Geometry check sheet. Reference: drawing and pictorial views, mm from the part's lowest x, y, z. A direction names the side the tool comes from. Round coordinates to 2 decimals unless told otherwise and drop trailing zeros. Loops run counter-clockwise (first coordinate to the right, second up) from the corner with the lowest first, then second, coordinate; pieces in that order, holes last. Notation, with made-up numbers: (-35.5, -29.75) -> (-1.5, -29.75) arc R20 cw to (-1.5, -14.75) -> close; hole circle Ø2 at (53, -25). An arc over 180 degrees is marked (long way). Use one line per item in the form item = value.
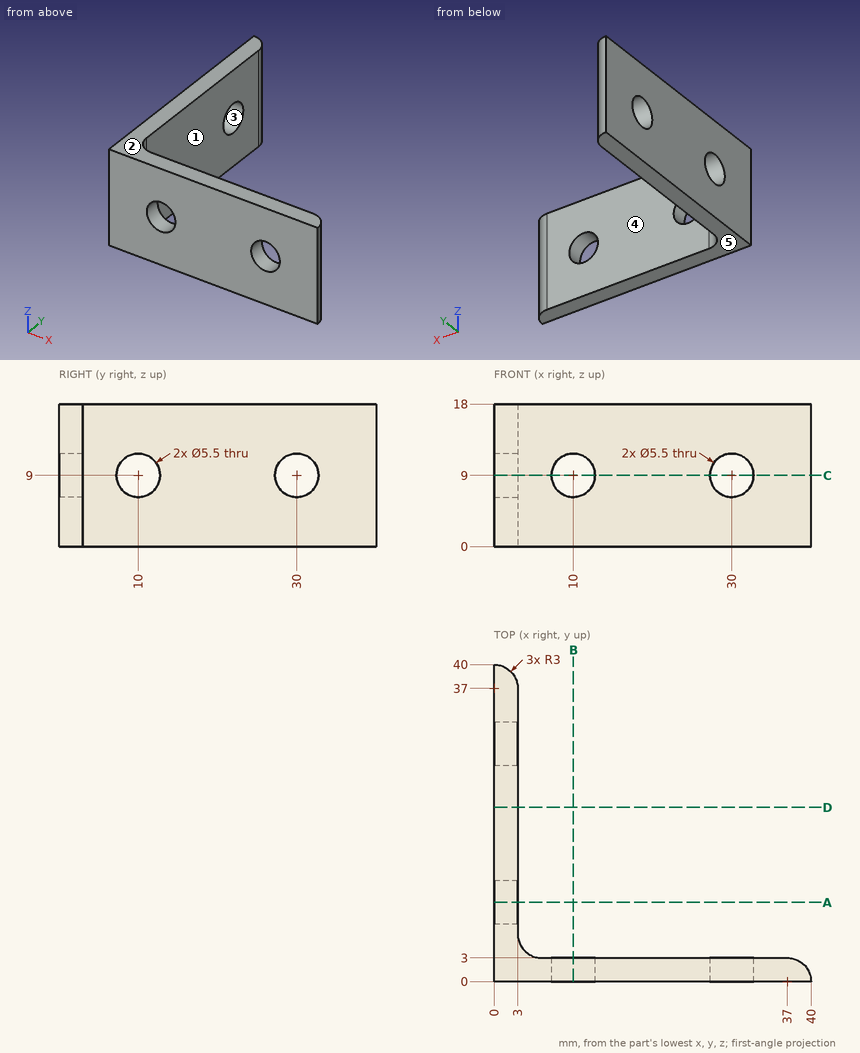
1. Section check D-D (y = 22). Record the boundary of the cut face in (x, z).
Return value:
outline = (0, 0) -> (3, 0) -> (3, 18) -> (0, 18) -> close
2. Section check A-A (y = 10). Record the boundary of the cut face in (x, z), then the cut area to 3 significant figures.
Return value:
outline = (0, 0) -> (3, 0) -> (3, 6.25) -> (0, 6.25) -> close; (0, 11.75) -> (3, 11.75) -> (3, 18) -> (0, 18) -> close
area = 37.5 mm2
3. Tool access check on the marked faces 1 and 2. Record the directions out of +Z, -Z, +X, -X, +Y, -Y that give a thin tool (end or side, any length) a straight path to the whole face; none if there is none.
Return value:
face_1 = +Z, -Z, +X, +Y
face_2 = +Z, +X, -X, +Y, -Y
4. Section check C-C (z = 9). Record the boundary of the cut face in (x, y), then the cut area to 3 significant figures.
Return value:
outline = (0, 0) -> (7.25, 0) -> (7.25, 3) -> (6, 3) arc R3 cw to (3, 6) -> (3, 7.25) -> (0, 7.25) -> close; (0, 12.75) -> (3, 12.75) -> (3, 27.25) -> (0, 27.25) -> close; (0, 32.75) -> (3, 32.75) -> (3, 37) arc R3 ccw to (0, 40) -> close; (12.75, 0) -> (27.25, 0) -> (27.25, 3) -> (12.75, 3) -> close; (32.75, 0) -> (40, 0) arc R3 ccw to (37, 3) -> (32.75, 3) -> close
area = 163 mm2
5. Gauge pin test, flat ends, axial feed: pin 1 (2 mm diameter, centred on x = 33, z = 6.5, fed in from +Y); pin 2 (5.5 mm diameter, centred on y = 14, z = 10.5, fed in from +X); pin 3 (4.5 mm diameter, centred on y = 30, z = 9, fed in from -X). Record the tip position at first contact, or that the pin passes through.
Return value:
pin_1 = 3
pin_2 = 3
pin_3 = through
6. Material ranges on line 1 along Y through (x, z) = (1.6, 9); line 2 along Y through (x, z) = (0.75, 9); line 3 along Y through (x, z) = (19.5, 7), recorded low to high.
Return value:
line_1 = 0 to 7.25, 12.75 to 27.25, 32.75 to 39.54
line_2 = 0 to 7.25, 12.75 to 27.25, 32.75 to 39.9
line_3 = 0 to 3
7. Mould release check, pull along Z, two halves, no side actions. Record for the marked faces 3, 4 and 5: released by +Z, released by -Z, zero draft, split by the parting line, or undercut.
Return value:
face_3 = undercut
face_4 = zero draft
face_5 = released by -Z
